Source: CAD feature listing. Evaluate the final solid. Frame: model axes, mm. Face numbers are marked on the shaded views. A direction names the side the tool comes from. Coordinates: 2 decimals unless noted, no trailing zeros. Order: outer loops, then holes, each group sorted by start corner. A loop starts at its lowest first (then second) coordinate and runs counter-clockwise, first axis right, second up.
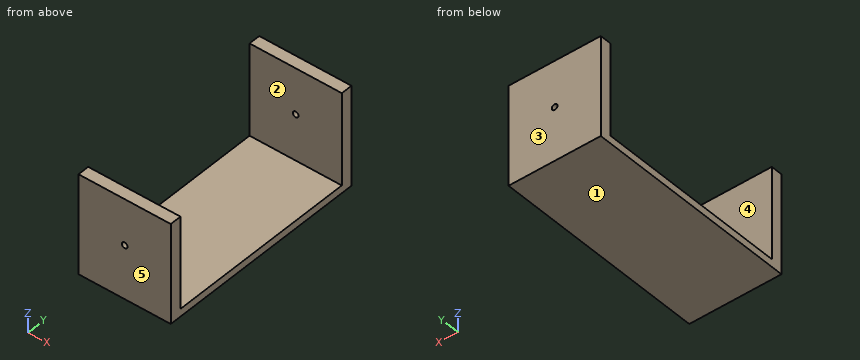
```python
from build123d import *

# Parameters (mm, degrees)
F0_W     = 19.05
F0_H     = 152.4
F0_H_2   = 12.7
F0_W_2   = 317.5
F1_DEPTH = 152.4
F2_R     = 4.7625
F3_DEPTH = 406.4


with BuildPart() as f1:
    # F0 (on Right) → F1 (new body)
    with BuildSketch(Plane.YZ):
        with Locations((9.525, 88.9)):
            Rectangle(F0_W, F0_H)
        with Locations((9.525, 6.35)):
            Rectangle(F0_W, F0_H_2)
        with Locations((177.8, 6.35)):
            Rectangle(F0_W_2, F0_H_2)
        with Locations((346.075, 88.9)):
            Rectangle(F0_W, F0_H)
        with Locations((346.075, 6.35)):
            Rectangle(F0_W, F0_H_2)
    extrude(amount=F1_DEPTH)

    # F2 (on Front) → F3 (cut)
    with BuildSketch(Plane.XZ):
        with Locations((76.2, 88.9)):
            Circle(F2_R)
    extrude(amount=-F3_DEPTH, mode=Mode.SUBTRACT)


solid = f1.part
```
1. Section query A-A on z = 88.9. Return loops of the section in (x, y).
Findings:
outline: (0, 0) - (71.44, 0) - (71.44, 19.05) - (0, 19.05) - close; (0, 336.55) - (71.44, 336.55) - (71.44, 355.6) - (0, 355.6) - close; (80.96, 0) - (152.4, 0) - (152.4, 19.05) - (80.96, 19.05) - close; (80.96, 336.55) - (152.4, 336.55) - (152.4, 355.6) - (80.96, 355.6) - close
2. Section query C-C on x = 111.5. Return loops of the section in (y, z), plus the area to 3 significant figures.
Findings:
outline: (0, 0) - (355.6, 0) - (355.6, 165.1) - (336.55, 165.1) - (336.55, 12.7) - (19.05, 12.7) - (19.05, 165.1) - (0, 165.1) - close
area: 10,300 mm2
3. Pin query (flat end, axial travel): P1, Ø5.5, axis at x = 76.2, z = 88.9, coming from the +Y side; P2, Ø1.5, axis at x = 33, y = 244.5, coming from the +Z side. Return the tip coordinate at first contact, or that it passes through.
Findings:
P1: passes through
P2: stops at z = 12.7
4. Section query B-B on x = 76.2. Return loops of the section in (y, z).
Findings:
outline: (0, 0) - (355.6, 0) - (355.6, 84.14) - (336.55, 84.14) - (336.55, 12.7) - (19.05, 12.7) - (19.05, 84.14) - (0, 84.14) - close; (0, 93.66) - (19.05, 93.66) - (19.05, 165.1) - (0, 165.1) - close; (336.55, 93.66) - (355.6, 93.66) - (355.6, 165.1) - (336.55, 165.1) - close
5. Draft query along Y for the marked faces 3, 4 and 5. Return one class per face: released by +Y, released by -Y, zero draft, split by the parting line, or undercut.
Findings:
face 3: released by +Y
face 4: undercut
face 5: released by -Y
6. Access query for the marked faces 1 and 2. Directions: +Z, -Z, +X, -X, +Y, -Y. A direction counts if a zero-diameter tool reaches every point of the face in a straight line with its end or side. Return the directions, or none.
Findings:
face 1: -Z, +X, -X, +Y, -Y
face 2: +Z, +X, -X
7. Section query D-D on y = 250.5. Return loops of the section in (x, z), plus the area to 3 significant figures.
Findings:
outline: (0, 0) - (152.4, 0) - (152.4, 12.7) - (0, 12.7) - close
area: 1,940 mm2
8. Ray query, line 1 (Y direction, x = 141, z = 24.5); line 2 (Z direction, x = 76.2, y = 11). Return the intervals inside material, ascending.
Findings:
line 1: y = 0 to 19.05, 336.55 to 355.6
line 2: z = 0 to 84.14, 93.66 to 165.1
